```python
from build123d import *

# Parameters (mm, degrees)
BOSS_EXTRUDE1_DEPTH = 90
FILLET1_R           = 1


with BuildPart() as part:
    # Sketch1 → Boss-Extrude1 (new body)
    with BuildSketch(Plane.XY):
        Polygon((-25, 0), (25, 0), (25, 15), (20, 15), (20, 10), (-20, 10), (-20, 15), (-25, 15), align=None)
    extrude(amount=BOSS_EXTRUDE1_DEPTH)

    # Fillet1
    fillet1_edges = [part.edges().sort_by_distance(p)[0] for p in [
        (-25, 15, 45),
        (25, 15, 45),
        (25, 0, 45),
        (-25, 0, 45),
    ]]
    fillet(fillet1_edges, radius=FILLET1_R)


solid = part.part
```
Geometry: final body of the model. Coordinates: model frame, mm. A direction names the side the tool comes from. Coordinates: 2 decimals unless noted, no trailing zeros. Order: outer loops, then holes, each group sorted by start corner. A loop starts at its lowest first (then second) coordinate and runs counter-clockwise, first axis right, second up. Notation, with made-up numbers: (14, 85.5) -> (26, 85.5) arc R15 cw to (26, 110.5) -> close; hole circle Ø8 at (68.25, 85). An arc over 180 degrees is marked (long way). Write item = value, one per line.
(1) Cut plane C-C on x = 11. Return loops of the section in (y, z).
Solved:
outline = (0, 0) -> (10, 0) -> (10, 90) -> (0, 90) -> close
(2) Pull-direction query (X, two-part tool) for faces 1 (the flat face through (25, 7, 44)), 2 (the flat face through (20, 13, 44)), 3 (the flat face through (0, 0, 44)), 4 (the flat face through (-20, 12, 44)); classes: pulls with the +X half, pulls with the -X half, needs draft (parallel to the pull), parting line crosses it, or undercut.
Solved:
face_1 = pulls with the +X half
face_2 = undercut
face_3 = needs draft
face_4 = undercut
(3) Cut plane B-B on z = 37. Return loops of the section in (x, y).
Solved:
outline = (-25, 1) arc R1 ccw to (-24, 0) -> (24, 0) arc R1 ccw to (25, 1) -> (25, 14) arc R1 ccw to (24, 15) -> (20, 15) -> (20, 10) -> (-20, 10) -> (-20, 15) -> (-24, 15) arc R1 ccw to (-25, 14) -> close
(4) Pin query (flat end, axial travel): pin 1 Ø1 at (x, y) = (-7, 8) entering from -Z; pin 2 Ø10 at (x, z) = (-4, 59.5) entering from +Y. Return the tip coordinate at first contact, or that it passes through.
Solved:
pin_1 = 0
pin_2 = 10
(5) Cut plane A-A on y = 12.75. Return loops of the section in (x, z), plus the area to 3 significant figures.
Solved:
outline = (-25, 0) -> (-20, 0) -> (-20, 90) -> (-25, 90) -> close; (20, 0) -> (25, 0) -> (25, 90) -> (20, 90) -> close
area = 900 mm²
(6) Line query: line 1 (X direction, y = 11.5, z = 46); line 2 (Y direction, x = -2.5, z = 66.5). Output: solid intervals per line, ascending.
Solved:
line_1 = -25 to -20, 20 to 25
line_2 = 0 to 10
(7) Access query for faces 5 (the flat face through (0, 10, 44)), 6 (the flat face through (0, 6, 90)). Directions: +Z, -Z, +X, -X, +Y, -Y. A direction counts if a zero-diameter tool reaches every point of the face in a straight line with its end or side. Return the directions, or none.
Solved:
face_5 = +Z, -Z, +Y
face_6 = +Z, +X, -X, +Y, -Y
